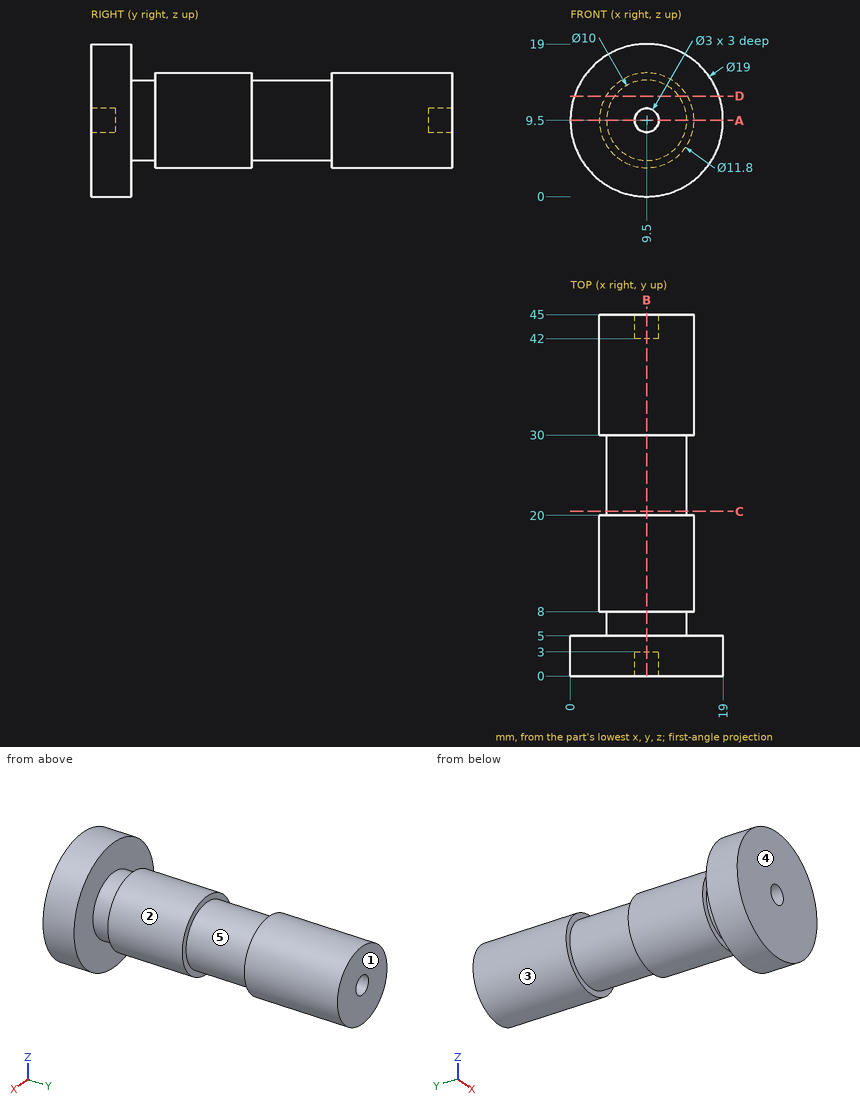
Part print with two shaded views. Sizes in mm from the minimum x, y, z corner. A direction names the side the tool comes from. Round coordinates to 2 decimals unless told otherwise and drop trailing zeros. Order: outer loops, then holes, each group sorted by start corner. A loop starts at its lowest first (then second) coordinate and runs counter-clockwise, first axis right, second up. Notation, with made-up numbers: M 85,38 L 108,38 A32 cw 108,73 Z; hole C 18,-24 d9. An arc over 180 degrees is marked long. Put each result on its own line as item: value. Start each with the question number.
1. Slice it at D-D on z = 12.5. List the corners of the cut face in (x, y).
2. Slice it at A-A on z = 9.5. List the corners of the cut face in (x, y).
3. Two-plate mould, pull along Y, no slides. Class the marked faces 3, 4 and 5: +Y half, -Y half, draft (parallel to the pull), parting line (faces both ways), or undercut.
4. Slice it at B-B on x = 9.5. List the corners of the cut face in (y, z).
5. Drop flat-ended pins along their axis: pin 1 (1 mm diameter, centred on y = 39, z = 12, fed in from -X); pin 2 (4 mm diameter, centred on y = 9.5, z = 10.5, fed in from -X); pin 3 (1.5 mm diameter, centred on x = 9.5, z = 10, fed in from -Y). Give the stop position or say it passes through.
6. Slice it at C-C on y = 20.5. List the corners of the cut face in (x, z), then the cut area to 3 significant figures.
7. Drill centre lines: probe 1 along Y at (x, z) = (12, 14.25); probe 2 along X at (y, z) = (44.3, 9.5); probe 3 along X at (y, z) = (0.95, 9.5). Where is each one in solid material? Low to high. Write a range as [from, to].
8. Tool access for the marked faces 1 and 2: list every direction of +Z, -Z, +X, -X, +Y, -Y with a clear straight run to the whole face (end or side of a thin tool).
Findings:
1. outline: M 0.49,0 L 18.51,0 L 18.51,5 L 13.5,5 L 13.5,8 L 14.58,8 L 14.58,20 L 13.5,20 L 13.5,30 L 14.58,30 L 14.58,45 L 4.42,45 L 4.42,30 L 5.5,30 L 5.5,20 L 4.42,20 L 4.42,8 L 5.5,8 L 5.5,5 L 0.49,5 Z
2. outline: M 0,0 L 8,0 L 8,3 L 11,3 L 11,0 L 19,0 L 19,5 L 14.5,5 L 14.5,8 L 15.4,8 L 15.4,20 L 14.5,20 L 14.5,30 L 15.4,30 L 15.4,45 L 11,45 L 11,42 L 8,42 L 8,45 L 3.6,45 L 3.6,30 L 4.5,30 L 4.5,20 L 3.6,20 L 3.6,8 L 4.5,8 L 4.5,5 L 0,5 Z
3. face 3: draft
3. face 4: -Y half
3. face 5: undercut
4. outline: M 0,0 L 5,0 L 5,4.5 L 8,4.5 L 8,3.6 L 20,3.6 L 20,4.5 L 30,4.5 L 30,3.6 L 45,3.6 L 45,8 L 42,8 L 42,11 L 45,11 L 45,15.4 L 30,15.4 L 30,14.5 L 20,14.5 L 20,15.4 L 8,15.4 L 8,14.5 L 5,14.5 L 5,19 L 0,19 L 0,11 L 3,11 L 3,8 L 0,8 Z
5. pin 1: x = 3.95
5. pin 2: x = 3.6
5. pin 3: y = 3
6. outline: C 9.5,9.5 d10
6. area: 78.5 mm2
7. probe 1: [0, 5], [8, 20], [30, 45]
7. probe 2: [3.6, 8], [11, 15.4]
7. probe 3: [0, 8], [11, 19]
8. face 1: +Z, -Z, +X, -X, +Y
8. face 2: +Y
